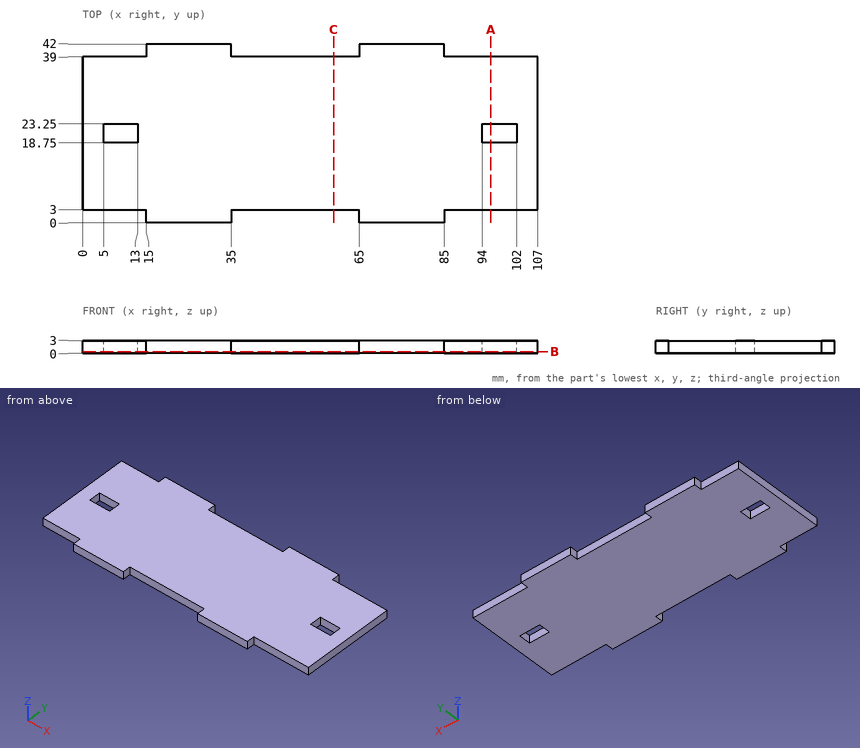
Geometry check sheet. Reference: drawing and pictorial views, mm from the part's lowest x, y, z. Round coordinates to 2 decimals unless told otherwise and drop trailing zeros. Write each loop counter-clockwise with the first axis right and the second up, starting at its lowest first coordinate (ties: lowest second). Pieces come first, ordered by that corner, then holes.
(1) Material ranges on line 1 (Y direction, x = 101, z = 1.75); line 2 (Y direction, x = 59.5, z = 1.8), recorded low to high.
Returned:
line 1: y = 3 to 18.75, 23.25 to 39
line 2: y = 3 to 39
(2) Section check A-A (x = 96). Enter the section's corners in (y, z).
Returned:
outline: (3, 0) - (18.75, 0) - (18.75, 3) - (3, 3) - close; (23.25, 0) - (39, 0) - (39, 3) - (23.25, 3) - close
(3) Section check C-C (x = 59). Enter the section's corners in (y, z), plus the area to 3 significant figures.
Returned:
outline: (3, 0) - (39, 0) - (39, 3) - (3, 3) - close
area: 108 mm2
(4) Section check B-B (z = 0.45). Enter the section's corners in (x, y).
Returned:
outline: (0, 3) - (15, 3) - (15, 0) - (35, 0) - (35, 3) - (65, 3) - (65, 0) - (85, 0) - (85, 3) - (107, 3) - (107, 39) - (85, 39) - (85, 42) - (65, 42) - (65, 39) - (35, 39) - (35, 42) - (15, 42) - (15, 39) - (0, 39) - close; hole (5, 18.75) - (13, 18.75) - (13, 23.25) - (5, 23.25) - close; hole (94, 18.75) - (102, 18.75) - (102, 23.25) - (94, 23.25) - close
(5) Depth check by flat-ended pin: pin 1 Ø1.5 at (y, z) = (40.5, 1) entering from -X; pin 2 Ø0.9 at (y, z) = (2, 1.5) entering from +X; pin 3 Ø0.9 at (x, z) = (100, 2) entering from +Y. Enter the tip coordinate at first touch or a pass-through.
Returned:
pin 1: stops at x = 15
pin 2: stops at x = 85
pin 3: stops at y = 39
